Answer from the drawing. Dimensions are ordinates in mm from the lowest x, y and z of the part. Round coordinates to 2 decimals unless told otherwise and drop trailing zeros. Order: outer loops, then holes, each group sorted by start corner. A loop starts at its lowest first (then second) coordinate and runs counter-clockwise, first axis right, second up.
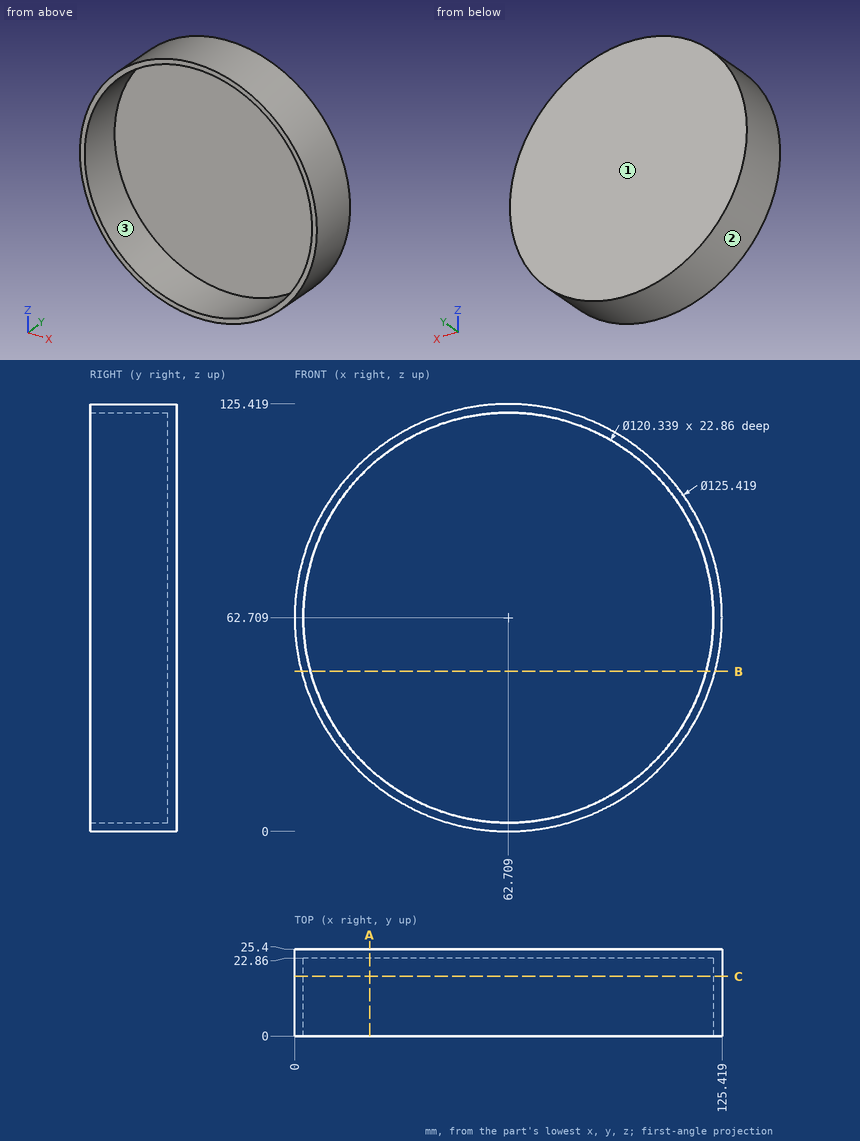
Q1. Flat-ended cylindrical pins translate along their axes: pin 1 (1 mm diameter, centred on y = 16.5, z = 76.5, fed in from -X) (1 decimal); pin 2 (3 mm diameter, centred on x = 48, z = 62.5, fed in from -Y); pin 3 (8 mm diameter, centred on y = 3, z = 98, fed in from -X) (1 decimal). Find the tip coordinate at first contact, or state that the pin passes through.
Outcome:
pin 1: stops at x = 1.4
pin 2: stops at y = 22.86
pin 3: stops at x = 8.4
Q2. A cutting plane is placed at B-B, the plane z = 47. Give the vertices of the cut face in (x, y).
Outcome:
outline: (2, 0) - (4.63, 0) - (4.63, 22.86) - (120.79, 22.86) - (120.79, 0) - (123.42, 0) - (123.42, 25.4) - (2, 25.4) - close
Q3. For a pull along X with two mould halves and no side action, classify the marked faces 1, 2 and 3 as released by +X, released by -X, zero draft, split by the parting line, or undercut.
Outcome:
face 1: zero draft
face 2: split by the parting line
face 3: undercut
Q4. A cutting plane is placed at A-A, the plane x = 22. Give the vertices of the cut face in (y, z).
Outcome:
outline: (0, 15.01) - (25.4, 15.01) - (25.4, 110.41) - (0, 110.41) - (0, 107.02) - (22.86, 107.02) - (22.86, 18.4) - (0, 18.4) - close
Q5. Straight lines are drawn through the part: probe 1 along X at (y, z) = (4.75, 63); probe 2 along Y at (x, z) = (68, 109). For each, find the intervals that lie inside material, in ascending order.
Outcome:
probe 1: x = 0 to 2.54, 122.88 to 125.42
probe 2: y = 22.86 to 25.4
Q6. A cutting plane is placed at C-C, the plane y = 17.5. Give the vertices of the cut face in (x, z).
Outcome:
outline: circle Ø125.42 at (62.71, 62.71); hole circle Ø120.34 at (62.71, 62.71)
